Geometry check sheet. Reference: the model listing, model coordinates, mm. A direction names the side the tool comes from. Coordinates: 2 decimals unless noted, no trailing zeros. Write each loop counter-clockwise with the first axis right and the second up, starting at its lowest first coordinate (ties: lowest second). Pieces come first, ordered by that corner, then holes. Notation, with made-up numbers: (8, 30) -> (20, 30) arc R14 ccw to (20, 38) -> close; hole circle Ø10 at (26.5, 4.5). An arc over 180 degrees is marked (long way). One line per question, with ' | ' between items.
```python
from build123d import *

# Parameters (mm, degrees)
SKETCH1_W           = 38.1
SKETCH1_H           = 25.4
SKETCH1_W_2         = 31.75
SKETCH1_H_2         = 19.05
BOSS_EXTRUDE1_DEPTH = 558.8
CUT_EXTRUDE1_REACH  = 561.701
SKETCH2_R           = 11.1125
SKETCH3_R           = 3.175
CUT_EXTRUDE2_DEPTH  = 3.175
SKETCH4_R           = 6.35
CUT_EXTRUDE3_DEPTH  = 3.175


with BuildPart() as part:
    # Sketch1 → Boss-Extrude1 (new body)
    with BuildSketch(Plane.XY):
        Rectangle(SKETCH1_W, SKETCH1_H)
        Rectangle(SKETCH1_W_2, SKETCH1_H_2, mode=Mode.SUBTRACT)
    extrude(amount=BOSS_EXTRUDE1_DEPTH)

    # Cut-Extrude1: up to this face of the body (flat: up to its plane)
    cut_extrude1_end = Plane(part.part.faces().sort_by_distance((0, -12.7, 279.4))[0])
    # Sketch2 → Cut-Extrude1 (cut, up to the picked face)
    with BuildSketch(Plane(origin=(0, 12.7, 0), x_dir=(1, 0, 0), z_dir=(0, 1, 0)), mode=Mode.PRIVATE) as cut_extrude1_sk1:
        with Locations(Location((0, -26.9875, 0), (0, 0, 270))):
            Circle(SKETCH2_R)
    cut_extrude1_tool1 = split(extrude(cut_extrude1_sk1.sketch, amount=-CUT_EXTRUDE1_REACH, mode=Mode.PRIVATE), bisect_by=cut_extrude1_end, keep=Keep.BOTH, mode=Mode.PRIVATE)
    add(cut_extrude1_tool1.solids().sort_by(Axis((0, 12.7, 26.9875), (0, -1, 0)))[0], mode=Mode.SUBTRACT)

    # Sketch3 → Cut-Extrude2 (cut)
    with BuildSketch(Plane.ZY.offset(19.05)):
        with Locations((538.1625, 0)):
            Circle(SKETCH3_R)
        with Locations((223.8375, 0)):
            Circle(SKETCH3_R)
    extrude(amount=-CUT_EXTRUDE2_DEPTH, mode=Mode.SUBTRACT)

    # Sketch4 → Cut-Extrude3 (cut)
    with BuildSketch(Plane(origin=(19.05, 0, 0), x_dir=(0, 0, -1), z_dir=(1, 0, 0))):
        with Locations((-538.1625, 0)):
            Circle(SKETCH4_R)
        with Locations((-223.8375, 0)):
            Circle(SKETCH4_R)
    extrude(amount=-CUT_EXTRUDE3_DEPTH, mode=Mode.SUBTRACT)


solid = part.part
```
(1) Cross-section at B-B (z = 367.5). Record the cut outline in (x, y) (3 decimals).
Answers below:
outline: (-19.05, -12.7) -> (19.05, -12.7) -> (19.05, 12.7) -> (-19.05, 12.7) -> close; hole (-15.875, -9.525) -> (15.875, -9.525) -> (15.875, 9.525) -> (-15.875, 9.525) -> close
(2) Tool access check on faces 1 (the face through (0, -9.525, 275)), 2 (the face through (17.48, 1.91, 217.78)), 3 (the face through (0, -11, 0)). Record the directions out of +Z, -Z, +X, -X, +Y, -Y that give a thin tool (end or side, any length) a straight path to the whole face; none if there is none.
Answers below:
face 1: +Z, -Z | face 2: +X | face 3: -Z, +X, -X, +Y, -Y
(3) Material ranges on line 1 (Y direction, x = -7.5, z = 98) (3 decimals); line 2 (X direction, y = 1.5, z = 407) (3 decimals); line 3 (Z direction, x = 17, y = -3.25), recorded low to high.
Answers below:
line 1: y = -12.7 to -9.525, 9.525 to 12.7 | line 2: x = -19.05 to -15.875, 15.875 to 19.05 | line 3: z = 0 to 218.38, 229.29 to 532.71, 543.62 to 558.8
(4) Draft check along Y on faces 4 (the face through (0, -12.7, 275)), 5 (the face through (0, -11, 558.8)), 6 (the face through (15.875, 0, 275)), 7 (the face through (17.485, 1.907, 532.106)). Enter one of: pulls with the +Y half, pulls with the -Y half, needs draft (parallel to the pull), parting line crosses it, or undercut.
Answers below:
face 4: pulls with the -Y half | face 5: needs draft | face 6: undercut | face 7: undercut
(5) Cross-section at A-A (x = 0). Record the cut outline in (y, z) (3 decimals).
Answers below:
outline: (-12.7, 0) -> (-9.525, 0) -> (-9.525, 15.875) -> (-12.7, 15.875) -> close; (-12.7, 38.1) -> (-9.525, 38.1) -> (-9.525, 558.8) -> (-12.7, 558.8) -> close; (9.525, 0) -> (12.7, 0) -> (12.7, 15.875) -> (9.525, 15.875) -> close; (9.525, 38.1) -> (12.7, 38.1) -> (12.7, 558.8) -> (9.525, 558.8) -> close
